```python
from build123d import *

# Parameters (mm, degrees)
F1_DEPTH = 3


with BuildPart() as f1:
    # F0 (on Top) → F1 (new body)
    with BuildSketch(Plane.XY):
        with BuildLine():
            Line((28.674154, 50.110632), (-31.325846, 50.110632))
            Line((-31.325846, 50.110632), (-31.325846, 47.110632))
            Line((-31.325846, 47.110632), (-33.840805, 47.110632))
            Line((-33.840805, 47.110632), (-54.905096, -43.760283))
            ThreePointArc((-54.905096, -43.760283), (-53.948671, -48.000202), (-50.034247, -49.889368))
            Line((-50.034247, -49.889368), (-45.299399, -49.889368))
            ThreePointArc((-45.299399, -49.889368), (-42.188565, -48.803792), (-40.42855, -46.018453))
            Line((-40.42855, -46.018453), (-26.692237, 13.239717))
            ThreePointArc((-26.692237, 13.239717), (-24.932222, 16.025056), (-21.821388, 17.110632))
            Line((-21.821388, 17.110632), (-1.5, 17.110632))
            Line((-1.5, 17.110632), (-1.5, 33.610632))
            Line((-1.5, 33.610632), (1.5, 33.610632))
            Line((1.5, 33.610632), (1.5, 17.110632))
            Line((1.5, 17.110632), (20.785474, 17.110632))
            ThreePointArc((20.785474, 17.110632), (23.94392, 15.986741), (25.682466, 13.120321))
            Line((25.682466, 13.120321), (37.85141, -45.899057))
            ThreePointArc((37.85141, -45.899057), (39.589956, -48.765477), (42.748401, -49.889368))
            Line((42.748401, -49.889368), (47.538051, -49.889368))
            ThreePointArc((47.538051, -49.889368), (51.414161, -48.047813), (52.435043, -43.879679))
            Line((52.435043, -43.879679), (33.674154, 47.110632))
            Line((33.674154, 47.110632), (28.674154, 47.110632))
            Line((28.674154, 47.110632), (28.674154, 50.110632))
        make_face()
    extrude(amount=F1_DEPTH)


solid = f1.part
```
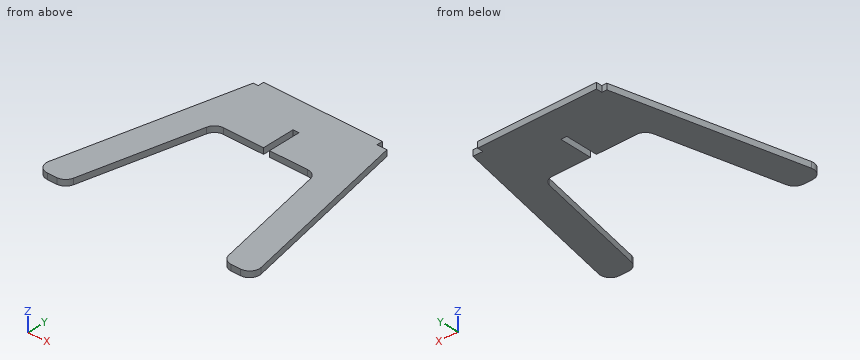
CAD build for the part. Positions are in the model's coordinates, mm. Coordinates: 2 decimals unless noted, no trailing zeros. Order: outer loops, then holes, each group sorted by start corner. A loop starts at its lowest first (then second) coordinate and runs counter-clockwise, first axis right, second up. Notation, with made-up numbers: (88.5, 16) - (137.5, 16) arc R33 ccw to (137.5, 52) - close; hole circle Ø7 at (20, 80.25). An arc over 180 degrees is marked (long way). Use a Markdown table: item, result. Add a question column.
(1) Saw through at D-D (y = 30.5). Give the cut face in (x, z), then the cut area to 3 significant figures.
(2) Flat gauge pins, fed straight in: pin 1 (1.5 mm diameter, centred on y = 49, z = 2, fed in from -X); pin 2 (0.8 mm diameter, centred on x = -32.5, z = 1, fed in from +Y); pin 3 (0.9 mm diameter, centred on x = -7.5, z = 1, fed in from -Y). Where does each tip first touch, or does it go through?
(3) Saw through at A-A (y = 7.5). Give the cut face in (x, z), then the cut area to 3 significant figures.
(4) Saw through at C-C (x = -19.5). Give the cut face in (y, z).
(5) Saw through at B-B (z = 1.75). Give the cut face in (x, y).
(6) Drill centre lines: line 1 along Y through (x, z) = (8, 1.95); line 2 along X through (y, z) = (-37.5, 1.7); line 3 along X through (y, z) = (20.5, 1.1). Where is each one in solid material? Low to high. Write a range as [from, to].
Solved:
| question | item | result |
|---|---|---|
| 1 | outline | (-37.69, 0) - (-1.5, 0) - (-1.5, 3) - (-37.69, 3) - close; (1.5, 0) - (37.1, 0) - (37.1, 3) - (1.5, 3) - close |
| 1 | area | 215 mm² |
| 2 | pin 1 | stops at x = -31.33 |
| 2 | pin 2 | stops at y = 47.11 |
| 2 | pin 3 | stops at y = 17.11 |
| 3 | outline | (-43.02, 0) - (-28.02, 0) - (-28.02, 3) - (-43.02, 3) - close; (26.84, 0) - (41.84, 0) - (41.84, 3) - (26.84, 3) - close |
| 3 | area | 90.0 mm² |
| 4 | outline | (17.11, 0) - (50.11, 0) - (50.11, 3) - (17.11, 3) - close |
| 5 | outline | (-54.91, -43.76) arc R5 ccw to (-50.03, -49.89) - (-45.3, -49.89) arc R5 ccw to (-40.43, -46.02) - (-26.69, 13.24) arc R5 cw to (-21.82, 17.11) - (-1.5, 17.11) - (-1.5, 33.61) - (1.5, 33.61) - (1.5, 17.11) - (20.79, 17.11) arc R5 cw to (25.68, 13.12) - (37.85, -45.9) arc R5 ccw to (42.75, -49.89) - (47.54, -49.89) arc R5 ccw to (52.44, -43.88) - (33.67, 47.11) - (28.67, 47.11) - (28.67, 50.11) - (-31.33, 50.11) - (-31.33, 47.11) - (-33.84, 47.11) - close |
| 6 | line 1 | y = [17.11, 50.11] |
| 6 | line 2 | x = [-53.45, -38.45], [36.12, 51.12] |
| 6 | line 3 | x = [-40.01, -1.5], [1.5, 39.16] |
